from build123d import *

# Parameters (mm, degrees)
F1_DEPTH = 50.8
F2_DEPTH = 50.8
F3_DEPTH = 50.8
F4_T     = 6.35
F5_R     = 6.35
F6_DEPTH = 114.301
F7_W     = 88.9
F7_H     = 50.8
F8_DEPTH = 58.7131


with BuildPart() as f1:
    # F0 (on Front) → F1 (new body, symmetric)
    with BuildSketch(Plane.XZ):
        with BuildLine():
            ThreePointArc((-52.3621, 0), (0, -52.3621), (52.3621, 0))
            ThreePointArc((52.3621, 0), (0, 52.3621), (-52.3621, 0))
        make_face()
    extrude(amount=F1_DEPTH, both=True)

    # F0 (on Front) → F2 (join)
    with BuildSketch(Plane.XZ):
        with BuildLine():
            ThreePointArc((-52.3621, 0), (0, 52.3621), (52.3621, 0))
            Line((52.3621, 0), (52.3621, 304.8))
            Line((52.3621, 304.8), (-52.3621, 304.8))
            Line((-52.3621, 304.8), (-52.3621, 0))
        make_face()
    extrude(amount=F2_DEPTH)

    # F0 (on Front) → F3 (join)
    with BuildSketch(Plane.XZ):
        with BuildLine():
            ThreePointArc((-52.3621, 0), (0, 52.3621), (52.3621, 0))
            Line((52.3621, 0), (52.3621, 304.8))
            Line((52.3621, 304.8), (-52.3621, 304.8))
            Line((-52.3621, 304.8), (-52.3621, 0))
        make_face()
    extrude(amount=-F3_DEPTH)

    # F4
    f4_openings = [f1.faces().sort_by_distance(p)[0] for p in [
        (0, 0, 304.8),
    ]]
    offset(amount=F4_T, openings=f4_openings, kind=Kind.INTERSECTION)

    # F5 (on face) → F6 (cut, through all)
    with BuildSketch(Plane.XZ.offset(57.15)):
        Circle(F5_R)
    extrude(amount=-F6_DEPTH, mode=Mode.SUBTRACT)

    # F7 (on Top) → F8 (cut, through all)
    with BuildSketch(Plane.XY):
        with Locations((1.5621, 0)):
            Rectangle(F7_W, F7_H)
    extrude(amount=-F8_DEPTH, mode=Mode.SUBTRACT)


solid = f1.part
The listing builds one solid part. Answer for the finished solid, in the listing's coordinates (mm). A direction names the side the tool comes from. Round coordinates to 2 decimals unless told otherwise and drop trailing zeros. Order: outer loops, then holes, each group sorted by start corner. A loop starts at its lowest first (then second) coordinate and runs counter-clockwise, first axis right, second up. Notation, with made-up numbers: M -17,57.25 L 32,57.25 A20 cw 32,65.25 Z; hole C -24,3 d4. An arc over 180 degrees is marked long. Answer in a Markdown table with one row per item. Add a question column.
1) Which of the six approach directions +Z, -Z, +X, -X, +Y, -Y give full straight-line access (tool end or side, diameter ignored) to faces 1 (the face through (46.012, 0, -31)), 2 (the face through (-1, -57.15, 126)), 3 (the face through (-1, 50.8, 129))?
2) The part is cut by section B-B on z = 137.5. Determine the outline of the cut face in (x, y), plus the area to 3 significant figures.
3) Consider line 1 along Y through (x, z) = (38, 16); line 2 along Z through (x, y) = (0, 55.75); line 3 along X through (y, z) = (-3, 151). Determine where each line is inside the solid, lowest interval first. Write a range as from..to.
4) The part is cut by section D-D on x = 23.5. Determine the outline of the cut face in (y, z).
5) Determine the mould class of faces 4 (the face through (-1.38, -54.02, -6.2)), 5 (the face through (-42.888, 0, -35)), 6 (the face through (-1.291, -26.2, -58.698)), 7 (the face through (-1.38, 53.93, -6.2)) for opening direction Z: pulls with the +Z half, pulls with the -Z half, needs draft (parallel to the pull), parting line crosses it, or undercut.
6) The part is cut by section C-C on x = 0. Determine the outline of the cut face in (y, z).
7) The part is cut by section A-A on y = 5.5. Determine the outline of the cut face in (x, z), plus the area to 3 significant figures.
8) Flat-ended cylindrical pins translate along their axes: pin 1 Ø3.5 at (y, z) = (8.5, -32) entering from -X; pin 2 Ø1.5 at (x, y) = (-20, -36.5) entering from -Z; pin 3 Ø8 at (x, y) = (28, -36.5) entering from +Z. Find the tip coordinate at first contact, or state that the pin passes through.
Findings below:
| question | item | result |
|---|---|---|
| 1 | face 1 | +Z, -Z |
| 1 | face 2 | +Z, -Z, +X, -X, -Y |
| 1 | face 3 | +Z |
| 2 | outline | M -58.71,-57.15 L 58.71,-57.15 L 58.71,57.15 L -58.71,57.15 Z; hole M -52.36,-50.8 L 52.36,-50.8 L 52.36,50.8 L -52.36,50.8 Z |
| 2 | area | 2,780 mm² |
| 3 | line 1 | y = -57.15..-50.8, 50.8..57.15 |
| 3 | line 2 | z = -58.71..-6.35, 6.35..304.8 |
| 3 | line 3 | x = -58.71..-52.36, 52.36..58.71 |
| 4 | outline | M -57.15,-53.8 L -25.4,-53.8 L -25.4,-46.79 L -50.8,-46.79 L -50.8,304.8 L -57.15,304.8 Z; M 25.4,-53.8 L 57.15,-53.8 L 57.15,304.8 L 50.8,304.8 L 50.8,-46.79 L 25.4,-46.79 Z |
| 5 | face 4 | undercut |
| 5 | face 5 | needs draft |
| 5 | face 6 | pulls with the -Z half |
| 5 | face 7 | undercut |
| 6 | outline | M -57.15,-58.71 L -25.4,-58.71 L -25.4,-52.36 L -50.8,-52.36 L -50.8,-6.35 L -57.15,-6.35 Z; M -57.15,6.35 L -50.8,6.35 L -50.8,304.8 L -57.15,304.8 Z; M 25.4,-58.71 L 57.15,-58.71 L 57.15,-6.35 L 50.8,-6.35 L 50.8,-52.36 L 25.4,-52.36 Z; M 50.8,6.35 L 57.15,6.35 L 57.15,304.8 L 50.8,304.8 Z |
| 7 | outline | M -58.71,0 A58.71 ccw -42.89,-40.1 L -42.89,-30.04 A52.36 cw -52.36,0 L -52.36,304.8 L -58.71,304.8 Z; M 46.01,-36.47 A58.71 ccw 58.71,0 L 58.71,304.8 L 52.36,304.8 L 52.36,0 A52.36 cw 46.01,-24.99 Z |
| 7 | area | 4,320 mm² |
| 8 | pin 1 | stops at x = -50.32 |
| 8 | pin 2 | stops at z = -55.47 |
| 8 | pin 3 | stops at z = -41.45 |
